Model file for the job. Use its own axes, mm. A direction names the side the tool comes from. Coordinates: 2 decimals unless noted, no trailing zeros. Write each loop counter-clockwise with the first axis right and the second up, starting at its lowest first coordinate (ties: lowest second). Pieces come first, ordered by that corner, then holes. Notation, with made-up numbers: M 82,82 L 88,82 A5 cw 88,90 Z; hole C 66.5,-2.5 d9. An arc over 180 degrees is marked long. One line per question, with ' | ' between items. Start each with the question number.
(1) Tool access for faces 1 (the face through (19, 17.879, -21)), 2 (the face through (55.872, 11.096, -20.716)), 3 (the face through (-22.99, 15.62, -0.05)), 4 (the face through (53.823, 2.218, 17.32)), 5 (the face through (58.733, 9.816, -0.454)): list every direction of +Z, -Z, +X, -X, +Y, -Y with a clear straight run to the whole face (end or side of a thin tool).
(2) Wall check: probe 1 along X at (y, z) = (2.5, 0) (1 decimal); probe 2 along X at (y, z) = (6.5, -0.5); probe 3 along Z at (x, y) = (18.5, 14.5). Give the ranges that are in metal, low to high.
(3) Two-plate mould, pull along Z, no slides. Class faces 6 (the face through (53.49, 2.22, -18.24)), 7 (the face through (-25.4, 9, 0)): +Z half, -Z half, draft (parallel to the pull), parting line (faces both ways), or undercut.
(4) Cut at C-C (x = 35). Write the cut outline in (y, z), plus the area to 3 significant figures.
(5) Flat gauge pins, fed straight in: pin 1 Ø6 at (x, z) = (57.15, -19.05) entering from -Y; pin 2 Ø5.5 at (x, z) = (-3.5, 0.5) entering from +Y; pin 3 Ø8 at (x, z) = (29, -6) entering from -Y. Where does each tip first touch, or does it go through?
(6) Cut at A-A (y = 11). Count the separate pieces of the cut face and the enclosed holes in it, plus the area to 3 significant figures.
from build123d import *

# Parameters (mm, degrees)
SKETCH1_R               = 15.875
SKETCH1_R_2             = 2.1
BOSS_EXTRUDE1_DEPTH     = 17.87906
CUT_EXTRUDE1_DEPTH      = 16.35506
SKETCH3_R               = 13.97
SKETCH3_R_2             = 8.89
BOSS_EXTRUDE2_DEPTH     = 0.254
SKETCH4_R               = 13.97
SKETCH4_R_2             = 10.99947
BOSS_EXTRUDE3_DEPTH     = 5.08
SKETCH5_R               = 17.399
SKETCH5_R_2             = 15.875
BOSS_EXTRUDE4_DEPTH     = 4.826
CUT_EXTRUDE2_REACH      = 96.17
CUT_EXTRUDE2_END_RADIUS = 20.6375
SKETCH6_R               = 2.2606
SKETCH7_R               = 3.75
CUT_EXTRUDE3_DEPTH      = 4.5


with BuildPart() as part:
    # Sketch1 → Boss-Extrude1 (new body)
    with BuildSketch(Plane(origin=(0, 0, 0), x_dir=(1, 0, 0), z_dir=(0, 1, 0))):
        with BuildLine():
            Line((-19.05, -25.4), (57.15, -25.4))
            ThreePointArc((57.15, -25.4), (61.640128061, -23.540128061), (63.5, -19.05))
            Line((63.5, -19.05), (63.5, 19.05))
            ThreePointArc((63.5, 19.05), (61.640128061, 23.540128061), (57.15, 25.4))
            Line((57.15, 25.4), (-19.05, 25.4))
            ThreePointArc((-19.05, 25.4), (-23.540128061, 23.540128061), (-25.4, 19.05))
            Line((-25.4, 19.05), (-25.4, -19.05))
            ThreePointArc((-25.4, -19.05), (-23.540128061, -23.540128061), (-19.05, -25.4))
        make_face()
        with Locations(Location((38.1, 0, 0), (0, 0, 270))):
            Circle(SKETCH1_R, mode=Mode.SUBTRACT)
        with Locations(Location((-19.05, 19.05, 0), (0, 0, 270))):
            Circle(SKETCH1_R_2, mode=Mode.SUBTRACT)
        with Locations(Location((-19.05, -19.05, 0), (0, 0, 270))):
            Circle(SKETCH1_R_2, mode=Mode.SUBTRACT)
        with Locations(Location((57.15, -19.05, 0), (0, 0, 270))):
            Circle(SKETCH1_R_2, mode=Mode.SUBTRACT)
        with Locations(Location((57.15, 19.05, 0), (0, 0, 270))):
            Circle(SKETCH1_R_2, mode=Mode.SUBTRACT)
    extrude(amount=BOSS_EXTRUDE1_DEPTH)

    # Sketch2 → Cut-Extrude1 (cut)
    with BuildSketch(Plane(origin=(0, 17.87906, 0), x_dir=(1, 0, 0), z_dir=(0, 1, 0))):
        with BuildLine():
            Line((0, 20.6375), (38.1, 20.6375))
            ThreePointArc((38.1, 20.6375), (58.7375, 0), (38.1, -20.6375))
            Line((38.1, -20.6375), (0, -20.6375))
            ThreePointArc((0, -20.6375), (-20.6375, 0), (0, 20.6375))
        make_face()
    extrude(amount=-CUT_EXTRUDE1_DEPTH, mode=Mode.SUBTRACT)

    # Sketch3 → Boss-Extrude2 (add)
    with BuildSketch(Plane(origin=(0, 1.524, 0), x_dir=(1, 0, 0), z_dir=(0, 1, 0))):
        with Locations(Location((0, 0, 0), (0, 0, 90))):
            Circle(SKETCH3_R)
        with Locations(Location((0, 0, 0), (0, 0, 270))):
            Circle(SKETCH3_R_2, mode=Mode.SUBTRACT)
    extrude(amount=BOSS_EXTRUDE2_DEPTH)

    # Sketch4 → Boss-Extrude3 (add)
    with BuildSketch(Plane(origin=(0, 1.778, 0), x_dir=(1, 0, 0), z_dir=(0, 1, 0))):
        with Locations(Location((0, 0, 0), (0, 0, 90))):
            Circle(SKETCH4_R)
        with Locations(Location((0, 0, 0), (0, 0, 270))):
            Circle(SKETCH4_R_2, mode=Mode.SUBTRACT)
    extrude(amount=BOSS_EXTRUDE3_DEPTH)

    # Sketch5 → Boss-Extrude4 (add)
    with BuildSketch(Plane(origin=(0, 1.524, 0), x_dir=(1, 0, 0), z_dir=(0, 1, 0))):
        with Locations(Location((38.1, 0, 0), (0, 0, 90))):
            Circle(SKETCH5_R)
        with Locations(Location((38.1, 0, 0), (0, 0, 270))):
            Circle(SKETCH5_R_2, mode=Mode.SUBTRACT)
    extrude(amount=BOSS_EXTRUDE4_DEPTH)

    # Cut-Extrude2: up to this cylinder (the profile starts outside it)
    cut_extrude2_end = Plane(origin=(0, 17.87906, 0), z_dir=(0, 1, 0)) * Cylinder(CUT_EXTRUDE2_END_RADIUS, 234.615, mode=Mode.PRIVATE)
    # Sketch6 → Cut-Extrude2 (cut, up to the surface)
    with BuildSketch(Plane.ZY.offset(25.4), mode=Mode.PRIVATE) as cut_extrude2_sk1:
        with Locations((0, 17.87906)):
            Circle(SKETCH6_R)
    cut_extrude2_tool1 = extrude(cut_extrude2_sk1.sketch, amount=-CUT_EXTRUDE2_REACH, mode=Mode.PRIVATE) - cut_extrude2_end
    add(cut_extrude2_tool1.solids().sort_by_distance((-25.4, 17.87906, 0))[0], mode=Mode.SUBTRACT)

    # Sketch7 → Cut-Extrude3 (cut)
    with BuildSketch(Plane.XZ):
        with Locations(Location((-19.05, 19.05, 0), (0, 0, 270))):
            Circle(SKETCH7_R)
        with Locations(Location((-19.05, -19.05, 0), (0, 0, 270))):
            Circle(SKETCH7_R)
        with Locations(Location((57.15, -19.05, 0), (0, 0, 270))):
            Circle(SKETCH7_R)
        with Locations(Location((57.15, 19.05, 0), (0, 0, 270))):
            Circle(SKETCH7_R)
    extrude(amount=-CUT_EXTRUDE3_DEPTH, mode=Mode.SUBTRACT)


solid = part.part
Filled in:
1) face 1: +Z, -Z, +X, -X, +Y | face 2: +Y, -Y | face 3: -X, +Y | face 4: -Y | face 5: +Y
2) probe 1: -25.4 to -20.6, -14 to -11, 11 to 14, 20.7 to 22.2, 54 to 55.5, 58.7 to 63.5 | probe 2: -25.4 to -20.63, -13.96 to -10.99, 10.99 to 13.96, 58.73 to 63.5 | probe 3: -25.4 to -20.64, 20.64 to 25.4
3) face 6: undercut | face 7: draft
4) outline: M 0,-25.4 L 17.88,-25.4 L 17.88,-20.64 L 1.52,-20.64 L 1.52,-17.12 L 6.35,-17.12 L 6.35,-15.57 L 0,-15.57 Z; M 0,15.57 L 6.35,15.57 L 6.35,17.12 L 1.52,17.12 L 1.52,20.64 L 17.88,20.64 L 17.88,25.4 L 0,25.4 Z | area: 201 mm²
5) pin 1: y = 4.5 | pin 2: y = 1.52 | pin 3: through
6) separate pieces: 1 | enclosed holes: 5 | area: 1,520 mm²
